from build123d import *

# Parameters (mm, degrees)
F0_R      = 200
F1_DEPTH  = 500
F2_R      = 60
F3_T      = -2.5
F6_DEPTH  = 644
F7_W      = 630.1204264164
F7_H      = 551.2289404869
F8_DEPTH  = 5
F12_DEPTH = 230
F16_DEPTH = 560.1
F19_DEPTH = 25


with BuildPart() as f1:
    # F0 (on Top) → F1 (new body)
    with BuildSketch(Plane.XY):
        Circle(F0_R)
    extrude(amount=F1_DEPTH)

    # F2
    f2_edges = [f1.edges().sort_by_distance(p)[0] for p in [
        (-200, 0, 0),
    ]]
    fillet(f2_edges, radius=F2_R)

    # F3
    f3_openings = [f1.faces().sort_by_distance(p)[0] for p in [
        (0, 0, 500),
    ]]
    offset(amount=F3_T, openings=f3_openings)

    # F5 (on offset) → F6 (join)
    with BuildSketch(Plane.XY.offset(200)):
        with BuildLine():
            ThreePointArc((199.311150361, 16.5850939631), (199.4115038067, -15.3314105532), (194.4334777301, -46.8574725929))
            Line((194.4334777301, -46.8574725929), (198.3221472847, -47.7946220448))
            ThreePointArc((198.3221472847, -47.7946220448), (203.3997338828, -15.6380387643), (203.2973733682, 16.9167958423))
            Line((203.2973733682, 16.9167958423), (199.311150361, 16.5850939631))
        make_face()
        with BuildLine():
            ThreePointArc((-16.5850939631, 199.311150361), (15.3314105532, 199.4115038067), (46.8574725929, 194.4334777301))
            Line((46.8574725929, 194.4334777301), (47.7946220448, 198.3221472847))
            ThreePointArc((47.7946220448, 198.3221472847), (15.6380387643, 203.3997338828), (-16.9167958423, 203.2973733682))
            Line((-16.9167958423, 203.2973733682), (-16.5850939631, 199.311150361))
        make_face()
        with BuildLine():
            ThreePointArc((-199.311150361, -16.5850939631), (-199.4115038067, 15.3314105532), (-194.4334777301, 46.8574725929))
            Line((-194.4334777301, 46.8574725929), (-198.3221472847, 47.7946220448))
            ThreePointArc((-198.3221472847, 47.7946220448), (-203.3997338828, 15.6380387643), (-203.2973733682, -16.9167958423))
            Line((-203.2973733682, -16.9167958423), (-199.311150361, -16.5850939631))
        make_face()
        with BuildLine():
            ThreePointArc((16.5850939631, -199.311150361), (-15.3314105532, -199.4115038067), (-46.8574725929, -194.4334777301))
            Line((-46.8574725929, -194.4334777301), (-47.7946220448, -198.3221472847))
            ThreePointArc((-47.7946220448, -198.3221472847), (-15.6380387643, -203.3997338828), (16.9167958423, -203.2973733682))
            Line((16.9167958423, -203.2973733682), (16.5850939631, -199.311150361))
        make_face()
    extrude(amount=-F6_DEPTH)

    # F7 (on face) → F8 (join)
    with BuildSketch(Plane(origin=(0, 0, -444), x_dir=(1, 0, 0), z_dir=(0, 0, -1))):
        with Locations((4.7718733549, -10.700315237)):
            Rectangle(F7_W, F7_H)
    extrude(amount=F8_DEPTH)

    # F11 (on 3pt) → F12 (cut)
    with BuildSketch(Plane(origin=(105.5092858466, -123.084311477, 0), x_dir=(-0.7592308548, -0.6508214111, 0), z_dir=(-0.6508214111, 0.7592308548, 0))):
        with BuildLine():
            ThreePointArc((-10, 87.8230258822), (0, 77.8230258822), (10, 87.8230258822))
            Line((10, 87.8230258822), (-10, 87.8230258822))
        make_face()
        with BuildLine():
            Line((-10, 87.8230258822), (10, 87.8230258822))
            ThreePointArc((10, 87.8230258822), (0, 97.8230258822), (-10, 87.8230258822))
        make_face()
    extrude(amount=-F12_DEPTH, mode=Mode.SUBTRACT)

    # F15 (on 3pt) → F16 (cut)
    with BuildSketch(Plane(origin=(-123.084311477, -105.5092858466, 0), x_dir=(-0.6508214111, 0.7592308548, 0), z_dir=(0.7592308548, 0.6508214111, 0))):
        with BuildLine():
            ThreePointArc((-10, 69.7543621063), (0, 59.7543621063), (10, 69.7543621063))
            Line((10, 69.7543621063), (-10, 69.7543621063))
        make_face()
        with BuildLine():
            Line((-10, 69.7543621063), (10, 69.7543621063))
            ThreePointArc((10, 69.7543621063), (0, 79.7543621063), (-10, 69.7543621063))
        make_face()
    extrude(amount=-F16_DEPTH, mode=Mode.SUBTRACT)

    # F18 (on offset) → F19 (join)
    with BuildSketch(Plane.XY.offset(108.5)):
        with BuildLine():
            ThreePointArc((-15.0850128449, 196.9230621016), (-0.1480075711, 197.4928535083), (14.789834964, 196.9454512847))
            ThreePointArc((14.789834964, 196.9454512847), (-0.1480128853, 197.4999445372), (-15.0850128449, 196.9230621016))
        make_face()
        with BuildLine():
            ThreePointArc((-162.9978679485, -111.5255353909), (-170.9598244185, -98.8746050706), (-177.9546814544, -85.6643528457))
            ThreePointArc((-177.9546814544, -85.6643528457), (-170.9659627725, -98.8781551874), (-162.9978679485, -111.5255353909))
        make_face()
        with BuildLine():
            ThreePointArc((163.1648464903, -111.281098439), (171.1139756579, -98.6217893498), (178.0828807935, -85.3975267107))
            ThreePointArc((178.0828807935, -85.3975267107), (171.1078319896, -98.6182484376), (163.1648464903, -111.281098439))
        make_face()
        with BuildLine():
            Line((-151.9739193408, -70.6643528457), (-177.9546814544, -85.6643528457))
            ThreePointArc((-177.9546814544, -85.6643528457), (-170.9598244185, -98.8746050706), (-162.9978679485, -111.5255353909))
            Line((-162.9978679485, -111.5255353909), (-137.0364954363, -96.5367299825))
            Line((-137.0364954363, -96.5367299825), (-151.9739193408, -70.6643528457))
        make_face()
        with BuildLine():
            ThreePointArc((163.1648464903, -111.281098439), (171.1078319896, -98.6182484376), (178.0828807935, -85.3975267107))
            Line((178.0828807935, -85.3975267107), (152.1215082813, -70.4087213022))
            Line((152.1215082813, -70.4087213022), (137.1840843768, -96.281098439))
            Line((137.1840843768, -96.281098439), (163.1648464903, -111.281098439))
        make_face()
        with BuildLine():
            Line((14.789834964, 166.9454512847), (14.789834964, 196.9454512847))
            ThreePointArc((14.789834964, 196.9454512847), (-0.1480075711, 197.4928535083), (-15.0850128449, 196.9230621016))
            Line((-15.0850128449, 196.9230621016), (-15.0850128449, 166.9454512847))
            Line((-15.0850128449, 166.9454512847), (14.789834964, 166.9454512847))
        make_face()
    extrude(amount=F19_DEPTH)


solid = f1.part
Build history of the part. All positions in model axes, mm. A direction names the side the tool comes from. Round coordinates to 2 decimals unless told otherwise and drop trailing zeros. Write each loop counter-clockwise with the first axis right and the second up, starting at its lowest first coordinate (ties: lowest second). Pieces come first, ordered by that corner, then holes. Notation, with made-up numbers: M 49.25,46 L 106.25,46 A33 ccw 106.25,78 Z; hole C 72.5,-2.5 d1. An arc over 180 degrees is marked long. Answer in a Markdown table with one row per item.
1. Saw through at C-C (x = 0). List the corners of the cut face in (y, z), and give its area (3 significant figures).
Geometry check:
| item | result |
|---|---|
| outline | M -264.91,-449 L 286.31,-449 L 286.31,-444 L 204,-444 L 204,200 L 200,200 L 200,500 L 197.5,500 L 197.5,133.5 L 166.95,133.5 L 166.95,108.5 L 197.5,108.5 L 197.5,60 A57.5 cw 140,2.5 L -140,2.5 A57.5 cw -197.5,60 L -197.5,500 L -200,500 L -200,200 L -204,200 L -204,-444 L -264.91,-444 Z; hole M -200,-444 L 200,-444 L 200,60 A60 cw 140,0 L -140,0 A60 cw -200,60 Z |
| area | 12,000 mm2 |
2. Saw through at D-D (z = 346). List the corners of the cut face in (x, y).
Geometry check:
| item | result |
|---|---|
| outline | C 0,0 d400; hole C 0,0 d395 |
3. Which spindle directions (+Z, -Z, +X, -X, +Y, -Y) get a long thin tool onto all of the face, cutting with end or side? Do faces 1 (the face through (0, 182, 108.5)), 2 (the face through (203.364, -16.093, -117.492)), 3 (the face through (-150.199, -104.136, 120.825)). Say none if no direction does.
Geometry check:
| item | result |
|---|---|
| face 1 | none |
| face 2 | +Z, +X |
| face 3 | +Z |
4. Saw through at A-A (z = -133.5). List the corners of the cut face in (x, y).
Geometry check:
| item | result |
|---|---|
| outline | M -203.3,-16.92 L -199.31,-16.59 A200 cw -194.43,46.86 L -198.32,47.79 A204 ccw Z; M -47.79,-198.32 A204 ccw 16.92,-203.3 L 16.59,-199.31 A200 cw -46.86,-194.43 Z; M -16.92,203.3 L -16.59,199.31 A200 cw 46.86,194.43 L 47.79,198.32 A204 ccw Z; M 194.43,-46.86 L 198.32,-47.79 A204 ccw 203.3,16.92 L 199.31,16.59 A200 cw Z |
5. Saw through at B-B (y = 0). List the corners of the cut face in (x, z), and give its area (3 significant figures).
Geometry check:
| item | result |
|---|---|
| outline | M -310.29,-449 L 319.83,-449 L 319.83,-444 L 204,-444 L 204,200 L 200,200 L 200,500 L 197.5,500 L 197.5,60 A57.5 cw 140,2.5 L -140,2.5 A57.5 cw -197.5,60 L -197.5,500 L -200,500 L -200,200 L -204,200 L -204,-444 L -310.29,-444 Z; hole M -200,-444 L 200,-444 L 200,60 A60 cw 140,0 L -140,0 A60 cw -200,60 Z |
| area | 11,700 mm2 |
6. Flat gauge pins, fed straight in: P1, Ø6, axis at x = -175.5, y = 17, coming from the +Z side; P2, Ø20.5, axis at x = -149, y = -89.5, coming from the +Z side; P3, Ø6, axis at x = 85.5, z = 166, coming from the +Y side. Where does each tip first touch, or does it go through?
Geometry check:
| item | result |
|---|---|
| P1 | z = 18.05 |
| P2 | z = 133.5 |
| P3 | y = 182.19 |
7. Mould opens along Z. For faces 4 (the face through (0, 7, -444)), 5 (the face through (157, -91, 133.5)), 6 (the face through (0, 166.945, 121)), 7 (the face through (157, -91, 108.5)) say: +Z half, -Z half, draft (parallel to the pull), parting line (faces both ways), or undercut.
Geometry check:
| item | result |
|---|---|
| face 4 | undercut |
| face 5 | +Z half |
| face 6 | draft |
| face 7 | undercut |
8. Probe L1, parallel to Z at x = -40.5, y = 44.5; L2, parallel to X at y = 0, z = 202. List the from-to ranges inside material, lowest first. Write a range as [from, to].
Geometry check:
| item | result |
|---|---|
| L1 | [-449, -444], [0, 2.5] |
| L2 | [-200, -197.5], [197.5, 200] |
